Could you check a few things on this drawing? It's one solid part, dimensions in mm from its lowest x, y, z. A direction names the side the tool comes from. Round coordinates to 2 decimals unless told otherwise and drop trailing zeros. Loops run counter-clockwise (first coordinate to the right, second up) from the corner with the lowest first, then second, coordinate; pieces in that order, holes last. Notation, with made-up numbers: (85, 13.5) -> (139, 13.5) arc R24 cw to (139, 32.5) -> close; hole circle Ø5 at (38, 62.25). An arc over 180 degrees is marked (long way). Use one line per item in the form item = value. Start each with the question number.
Item 1: Thinking about a two-plate mould opening in Y: for the marked faces 1, 2 and 3, which applies, released by +Y, released by -Y, zero draft, split by the parting line, or undercut?
Item 2: If I drill on L1, parallel to Y at x = 87.65, z = 19.85; L2, parallel to Y at x = 94.5, z = 12, over which ranges is the centre line in solid material (lowest first)? Write a range as [from, to].
Item 3: If we section it at B-B (x = 90): Write out the boundary of the cut face in (y, z).
Item 4: I'm going to push a flat-ended pin straight in: pin 1 Ø6 at (y, z) = (9, 14.5) entering from -X. Where does the tip first touch, or does it pass through?
Item 5: If we section it at A-A (z = 13.75): Write out the boundary of the cut face in (x, y).
Item 6: If we section it at D-D (y = 5): Write out the boundary of the cut face in (x, z).
Item 7: For the marked faces 4 and 5, which set-ups out of +Z, -Z, +X, -X, +Y, -Y let a thin tool reach every point of the face, with its end or its side?
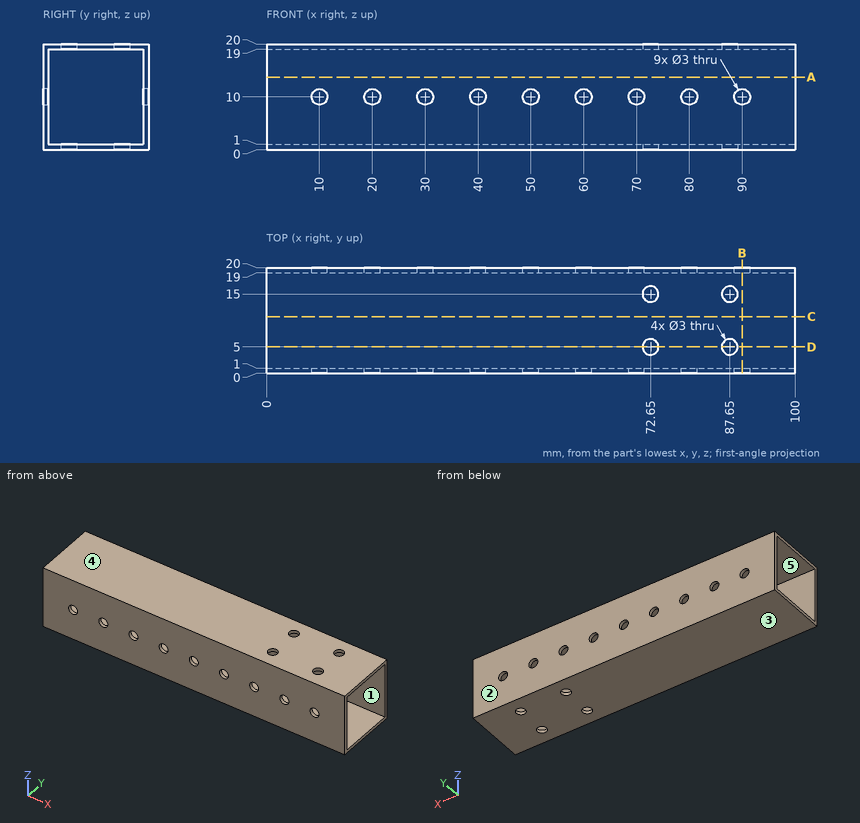
Values found:
q1.face_1 = undercut
q1.face_2 = released by +Y
q1.face_3 = zero draft
q2.L1 = [0, 3.5], [6.5, 13.5], [16.5, 20]
q2.L2 = [0, 1], [19, 20]
q3.outline = (0, 0) -> (20, 0) -> (20, 8.5) -> (19, 8.5) -> (19, 1) -> (1, 1) -> (1, 8.5) -> (0, 8.5) -> close; (0, 11.5) -> (1, 11.5) -> (1, 19) -> (19, 19) -> (19, 11.5) -> (20, 11.5) -> (20, 20) -> (0, 20) -> close
q4.pin_1 = through
q5.outline = (0, 0) -> (100, 0) -> (100, 1) -> (0, 1) -> close; (0, 19) -> (100, 19) -> (100, 20) -> (0, 20) -> close
q6.outline = (0, 0) -> (71.15, 0) -> (71.15, 1) -> (0, 1) -> close; (0, 19) -> (71.15, 19) -> (71.15, 20) -> (0, 20) -> close; (74.15, 0) -> (86.15, 0) -> (86.15, 1) -> (74.15, 1) -> close; (74.15, 19) -> (86.15, 19) -> (86.15, 20) -> (74.15, 20) -> close; (89.15, 0) -> (100, 0) -> (100, 1) -> (89.15, 1) -> close; (89.15, 19) -> (100, 19) -> (100, 20) -> (89.15, 20) -> close
q7.face_4 = +Z, +X, -X, +Y, -Y
q7.face_5 = +X, -X
